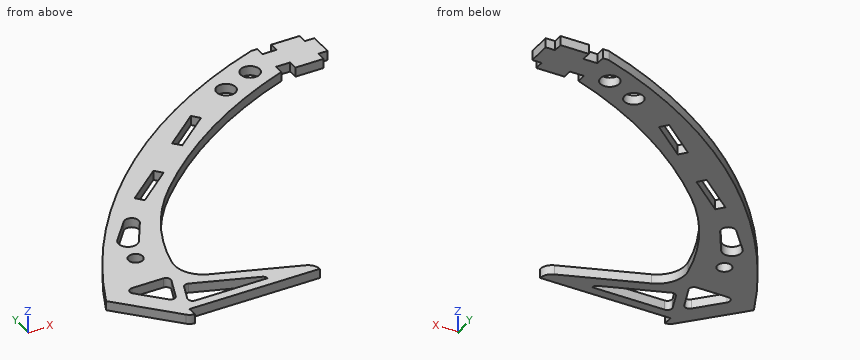
```python
from build123d import *

# Parameters (mm, degrees)
SKETCH1_R           = 1.5
SKETCH1_R_2         = 2
BOSS_EXTRUDE1_DEPTH = 2


with BuildPart() as part:
    # Sketch1 → Boss-Extrude1 (new body)
    with BuildSketch(Plane.XY):
        with BuildLine():
            Line((-62.309511, 0), (-90, 0))
            Line((-90, 0), (-90, -2))
            ThreePointArc((-90, -2), (-90.800086058, -1.832992717), (-91.466551917, -1.3598623))
            Line((-91.466551917, -1.3598623), (-102, 10))
            ThreePointArc((-102, 10), (-75.5606337, 47.428438735), (-36.262928729, 71))
            Line((-36.262928729, 71), (-35, 71))
            Line((-35, 71), (-35, 69))
            Line((-35, 69), (-32, 69))
            Line((-32, 69), (-32, 71))
            Line((-32, 71), (-26, 71))
            Line((-26, 71), (-26, 69))
            Line((-26, 69), (-24, 69))
            Line((-24, 69), (-24, 64))
            Line((-24, 64), (-26, 64))
            Line((-26, 64), (-26, 62))
            Line((-26, 62), (-32, 62))
            Line((-32, 62), (-32, 64))
            Line((-32, 64), (-35, 64))
            Line((-35, 64), (-35, 62))
            ThreePointArc((-35, 62), (-55.195926155, 51.990753781), (-72.706011232, 37.797186092))
            ThreePointArc((-72.706011232, 37.797186092), (-80.350726752, 27.513864966), (-84.859723335, 15.519811498))
            ThreePointArc((-84.859723335, 15.519811498), (-84.266660534, 11.330126172), (-81.056134593, 8.573731826))
            Line((-81.056134593, 8.573731826), (-63.954460642, 2.349231552))
            ThreePointArc((-63.954460642, 2.349231552), (-62.76163089, 1.433941091), (-62.309511, 0))
        make_face()
        with Locations((-90, 20)):
            Circle(SKETCH1_R, mode=Mode.SUBTRACT)
        with Locations((-46.864489858, 61.785493015)):
            Circle(SKETCH1_R_2, mode=Mode.SUBTRACT)
        with Locations((-39.993861134, 64.851566266)):
            Circle(SKETCH1_R_2, mode=Mode.SUBTRACT)
        with BuildLine():
            Line((-89.810992251, 27.099684807), (-85.686951519, 31.9596162))
            ThreePointArc((-85.686951519, 31.9596162), (-83.665127869, 32.205193808), (-83.262186445, 30.208767641))
            Line((-83.262186445, 30.208767641), (-86.577972152, 24.765220061))
            ThreePointArc((-86.577972152, 24.765220061), (-89.456863792, 24.184169423), (-89.810992251, 27.099684807))
        make_face(mode=Mode.SUBTRACT)
        with BuildLine():
            Line((-72.886250096, 2.939692621), (-85.819268287, 7.646926281))
            ThreePointArc((-85.819268287, 7.646926281), (-86.572995727, 7.618549798), (-87.092498654, 7.071716197))
            Line((-87.092498654, 7.071716197), (-88.543537199, 3.364482536))
            ThreePointArc((-88.543537199, 3.364482536), (-88.438305951, 2.436299076), (-87.612326975, 2))
            Line((-87.612326975, 2), (-72.228270239, 2))
            ThreePointArc((-72.228270239, 2), (-72.409118195, 2.573576436), (-72.886250096, 2.939692621))
        make_face(mode=Mode.SUBTRACT)
        with BuildLine():
            Line((-95.644910389, 11.5), (-88.972257251, 11.5))
            ThreePointArc((-88.972257251, 11.5), (-88.146278275, 11.063700924), (-88.041047027, 10.135517464))
            Line((-88.041047027, 10.135517464), (-90.021639474, 5.075335561))
            ThreePointArc((-90.021639474, 5.075335561), (-90.766646985, 4.457306749), (-91.686125656, 4.759886947))
            Line((-91.686125656, 4.759886947), (-96.378186348, 9.82006885))
            ThreePointArc((-96.378186348, 9.82006885), (-96.561406748, 10.900043029), (-95.644910389, 11.5))
        make_face(mode=Mode.SUBTRACT)
        Polygon((-78.661971859, 36.409830161), (-71.001527428, 42.837706258), (-72.287102647, 44.369795144), (-79.947547078, 37.941919047), align=None, mode=Mode.SUBTRACT)
        Polygon((-63.341082997, 49.265582354), (-64.626658216, 50.797671241), (-56.966213785, 57.225547337), (-55.680638565, 55.693458451), align=None, mode=Mode.SUBTRACT)
    extrude(amount=BOSS_EXTRUDE1_DEPTH)


solid = part.part
```
Read the model definition and answer for the solid it produces. Units are mm, in the model's axes. Give positions to 0.01 mm unless a question says otherwise; leave off trailing zeros. Loops run counter-clockwise (first coordinate to the right, second up) from the corner with the lowest first, then second, coordinate; pieces in that order, holes last.
Item 1: The part is cut by section D-D (z = 1.15). Give the number of separate pieces and of enclosed holes in the cut face, and give its area (3 significant figures).
Item 2: The part is cut by section A-A (x = -66.5). Write down the section's boundary in (y, z), and give its area (3 significant figures).
Item 3: The part is cut by section C-C (x = -29.5). Write down the section's boundary in (y, z), and give its area (3 significant figures).
Item 4: The part is cut by section B-B (y = 20). Write down the section's boundary in (x, z), and give its area (3 significant figures).
Item 5: Each of these flat-tipped pins is pushed along its axis until it touches: pin 1 Ø5 at (x, y) = (-90, 20) entering from +Z; pin 2 Ø1 at (y, z) = (63, 0.5) entering from +X; pin 3 Ø1 at (y, z) = (43.5, 1) entering from -X; pin 4 Ø1 at (x, z) = (-30, 0.5) entering from -Y. Where does it stop, or does it pass through?
Item 6: Find the intervals of material crossed by line 1 along Y through (x, z) = (-72, 0.2); line 2 along Y through (x, z) = (-68, 1.7); line 3 along Y through (x, z) = (-40, 1.75), in increasing order.
Taken from the geometry:
1. separate pieces: 1
1. enclosed holes: 8
1. area: 984 mm2
2. outline: (0, 0) - (3.28, 0) - (3.28, 2) - (0, 2) - close; (43.58, 0) - (54.98, 0) - (54.98, 2) - (43.58, 2) - close
2. area: 29.4 mm2
3. outline: (62, 0) - (71, 0) - (71, 2) - (62, 2) - close
3. area: 18.0 mm2
4. outline: (-97.08, 0) - (-91.5, 0) - (-91.5, 2) - (-97.08, 2) - close; (-88.5, 0) - (-83.62, 0) - (-83.62, 2) - (-88.5, 2) - close
4. area: 20.9 mm2
5. pin 1: stops at z = 2
5. pin 2: stops at x = -26
5. pin 3: stops at x = -80.07
5. pin 4: stops at y = 62
6. line 1: y = 0 to 5.28, 38.51 to 42, 44.03 to 50.59
6. line 2: y = 0 to 3.82, 42.27 to 53.84
6. line 3: y = 60.03 to 62.85, 66.85 to 69.63
